Autodesk Inventor part; units mm, degrees
ref_plane "Work Plane1" through (0, 0, 60) normal (0, 0, -1) x (-1, 0, 0)
ref_plane "Work Plane2" through (0, 0, 192) normal (0, 0, -1) x (-1, 0, 0)
ref_plane "Work Plane3" through (0, -25.1413, 0) normal (-1, 0, 0) x (0, 0, 1)
sketch "Sketch1" plane through (0, 0, 0) normal (0, 0, 1) x (1, 0, 0)
  line L0 (0, 0) -> (-20.6965, 9.6509) construction
  line L1 (0, 0) -> (0, -60.6509) construction
  line L2 (0, 0) -> (-23.2307, -49.8183) construction
  line L3 (0, 0) -> (21.0241, 9.8037) construction
  line L4 (0, 0) -> (21.5225, -46.1553) construction
  line L5 (0, 0) -> (0, 48) construction
  arc A0 (-36, -19.5) -> (36, -19.5) centre (0, 48) ccw
  line L6 (-36, -19.5) -> (-36, -25.1413)
  line L7 (36, -19.5) -> (36, -25.1413)
  line L8 (-10, -40.5) -> (10, -40.5)
  line L9 (-10, -40.5) -> (-10, -37.2653)
  line L10 (10, -40.5) -> (10, -37.2653)
  line L11 (-17.6908, -33.679) -> (-16.0004, -30.0538)
  line L12 (-16.0004, -30.0538) -> (-12.7377, -31.5752)
  line L13 (-12.7377, -31.5752) -> (-14.4281, -35.2004)
  line L14 (14.4281, -35.2004) -> (12.7377, -31.5752)
  line L15 (12.7377, -31.5752) -> (16.0004, -30.0538)
  line L16 (16.0004, -30.0538) -> (17.6908, -33.679)
  line L17 (10, -37.2653) -> (14.4281, -35.2004)
  line L18 (17.6908, -33.679) -> (36, -25.1413)
  line L19 (-10, -37.2653) -> (-14.4281, -35.2004)
  line L20 (-17.6908, -33.679) -> (-36, -25.1413)
  dimension "d0" = 25
  dimension "d1" = 90
  dimension "d2" = 90
  dimension "d3" = 25
  dimension "d4" = 48
  dimension "d5" = 153
  dimension "d11" = 72
  dimension "d12" = 36
  dimension "d13" = 20
  dimension "d14" = 10
  dimension "d17" = 88.5
  dimension "d18" = 3.6
  dimension "d19" = 1.8
  dimension "d20" = 4
  dimension "d21" = 1.8
  dimension "d22" = 1.8
  dimension "d23" = 4
extrude "Extrusion1" add sketch "Sketch1" along normal blind 325
ref_plane "Work Plane1" through (0, 0, 60) normal (0, 0, -1) x (-1, 0, 0)
sketch "Sketch2" plane through (0, 0, 60) normal (0, 0, -1) x (-1, 0, 0)
  line L0 (14.4281, -35.2004) -> (12.7377, -31.5752)
  line L1 (12.7377, -31.5752) -> (16.0004, -30.0538)
  line L2 (14.4281, -35.2004) -> (10, -37.2653)
  line L3 (16.0004, -30.0538) -> (25.4652, -30.0538)
  line L4 (25.4652, -30.0538) -> (14.4281, -35.2004)
  line L5 (12.7377, -31.5752) -> (14.4281, -35.2004)
  line L6 (16.0004, -30.0538) -> (12.7377, -31.5752)
  line L7 (36, -25.1413) -> (17.6908, -33.679)
  line L8 (10, -40.5) -> (-10, -40.5)
  line L9 (-14.4281, -35.2004) -> (-12.7377, -31.5752)
  line L10 (-12.7377, -31.5752) -> (-16.0004, -30.0538)
  line L11 (-16.0004, -30.0538) -> (-25.4652, -30.0538)
  line L12 (-25.4652, -30.0538) -> (-14.4281, -35.2004)
  line L13 (-14.4281, -35.2004) -> (-12.7377, -31.5752)
  line L14 (-12.7377, -31.5752) -> (-16.0004, -30.0538)
  line L15 (-10, -37.2653) -> (-14.4281, -35.2004)
  line L16 (-17.6908, -33.679) -> (-36, -25.1413)
  point P0 (0, 0)
extrude "Extrusion2" cut sketch "Sketch2" against normal blind 72
ref_plane "Work Plane2" through (0, 0, 192) normal (0, 0, -1) x (-1, 0, 0)
sketch "Sketch3" plane through (0, 0, 192) normal (0, 0, -1) x (-1, 0, 0)
  line L0 (14.4281, -35.2004) -> (12.7377, -31.5752)
  line L1 (12.7377, -31.5752) -> (14.4281, -35.2004)
  line L2 (12.7377, -31.5752) -> (16.0004, -30.0538)
  line L3 (16.0004, -30.0538) -> (25.4652, -30.0538)
  line L4 (25.4652, -30.0538) -> (14.4281, -35.2004)
  line L5 (-14.4281, -35.2004) -> (-12.7377, -31.5752)
  line L6 (-12.7377, -31.5752) -> (-16.0004, -30.0538)
  line L7 (-16.0004, -30.0538) -> (-25.4652, -30.0538)
  line L8 (-25.4652, -30.0538) -> (-14.4281, -35.2004)
  line L9 (16.0004, -30.0538) -> (12.7377, -31.5752)
  line L10 (14.4281, -35.2004) -> (10, -37.2653)
  line L11 (-14.4281, -35.2004) -> (-12.7377, -31.5752)
  line L12 (-12.7377, -31.5752) -> (-16.0004, -30.0538)
  line L13 (-10, -37.2653) -> (-14.4281, -35.2004)
  line L14 (10, -40.5) -> (-10, -40.5)
  line L15 (36, -25.1413) -> (17.6908, -33.679)
  point P0 (0, 0)
extrude "Extrusion3" cut sketch "Sketch3" against normal blind 73
ref_plane "Work Plane3" through (0, -25.1413, 0) normal (-1, 0, 0) x (0, 0, 1)
sketch "Sketch5" plane through (0, -25.1413, 0) normal (-1, 0, 0) x (0, 0, 1)
  line L0 (0, -7.5587) -> (0, -3.3587)
  line L1 (68, -7.5587) -> (68, -15.3587)
  line L2 (68, -15.3587) -> (138.7768, -15.3587)
  line L3 (138.7768, -15.3587) -> (108, -5.3587)
  line L4 (108, -5.3587) -> (108, -3.3587)
  line L5 (0, -15.3587) -> (325, -15.3587)
  line L6 (246, -7.5587) -> (246, -15.3587)
  line L7 (246, -15.3587) -> (316.7768, -15.3587)
  line L8 (68, -7.5587) -> (0, -7.5587)
  line L9 (286, -3.3587) -> (286, -5.3587)
  line L10 (316.7768, -15.3587) -> (286, -5.3587)
  line L11 (0, -3.3587) -> (0, -0.3587)
  line L12 (0, -8.5377) -> (0, 0)
  line L13 (0, 5.6413) -> (325, 5.6413)
  line L14 (286, -0.3587) -> (286, -3.3587)
  line L15 (246, -7.5587) -> (148, -7.5587)
  line L16 (148, -7.5587) -> (148, -3.3587)
  line L17 (108, -0.3587) -> (108, -3.3587)
  line L18 (325, -3.3587) -> (0, -3.3587)
  line L19 (148, -3.3587) -> (148, -0.3587)
  line L20 (0, -3.3587) -> (108, -3.3587)
  line L21 (148, -3.3587) -> (286, -3.3587)
  line L22 (0, -0.3587) -> (108, -0.3587)
  line L23 (148, -0.3587) -> (286, -0.3587)
  point P0 (0, 25.1413)
  dimension "d51" = 4.2
  dimension "d52" = 0
  dimension "d53" = 68
  dimension "d54" = 2
  dimension "d56" = 40
  dimension "d59" = 246
  dimension "d64" = 18
  dimension "d65" = 2
  dimension "d68" = 3
  dimension "d69" = 40
  dimension "d84" = 178
  dimension "d94" = 18
  dimension "d96" = 40
extrude "Extrusion4" cut sketch "Sketch5" along normal mid plane 6.5 contours L0 L18 L4 L3 L2 L1 L8 | L11 L22 L17 L18 | L18 L9 L10 L5 L6 L15 L16 | L19 L23 L14 L18
sketch "Sketch6" plane through (-10, -40.5, 0) normal (0, -1, 0) x (1, 0, 0)
  line L0 (-49, 178) -> (79, 178) construction
  line L1 (10, 0) -> (10, 369) construction
  arc A0 (11, 159) -> (11, 169) centre (11, 164) ccw
  arc A1 (16, 183) -> (16, 173) centre (16, 178) ccw
  line L2 (11, 159) -> (11, 169)
  line L3 (16, 173) -> (16, 183)
  line L4 (11, 187) -> (11, 197)
  arc A2 (11, 187) -> (11, 197) centre (11, 192) ccw
  point P0 (4, 178)
  dimension "d70" = 178
  dimension "d85" = 1
  dimension "d86" = 5
  dimension "d87" = 5
  dimension "d88" = 6
  dimension "d89" = 5
  dimension "d90" = 1
  dimension "d91" = 14
  dimension "d92" = 14
extrude "Extrusion5" add sketch "Sketch6" along normal blind 7
equation "\"BendRadius\" = Thickness"
equation "\"BendReliefWidth\" = Thickness"
equation "\"BendReliefDepth\" = 0.5 * Thickness"
equation "\"CornerReliefSize\" = 4 * Thickness"
equation "\"MinimumRemnant\" = 2 * Thickness"
equation "\"TransitionRadius\" = BendRadius"
equation "\"JacobiRadiusSize\" = BendRadius"
equation "\"GapSize\" = Thickness"
properties part number "3213_Bed Holder" material "Acetal Resin, White"
Work out the finished part from the listing and answer in its coordinate system (mm). A direction names the side the tool comes from. Coordinates: 2 decimals unless noted, no trailing zeros. Write each loop counter-clockwise with the first axis right and the second up, starting at its lowest first coordinate (ties: lowest second). Pieces come first, ordered by that corner, then holes. Notation, with made-up numbers: M 53.25,-35 L 86.25,-35 A23 cw 86.25,0 Z; hole C 74.25,68.25 d11. An arc over 180 degrees is marked long. Write item = value, one per line.
1. The part is cut by section D-D (z = 164). Determine the outline of the cut face in (x, y), then the cut area to 3 significant figures.
Solution:
outline = M -36,-25.14 L -17.69,-33.68 L -16,-30.05 L -12.74,-31.58 L -14.43,-35.2 L -10,-37.27 L -10,-40.5 L 1,-40.5 L 1,-47.5 L 6,-47.5 L 6,-40.5 L 10,-40.5 L 10,-37.27 L 14.43,-35.2 L 12.74,-31.58 L 16,-30.05 L 17.69,-33.68 L 36,-25.14 L 36,-19.5 A76.5 cw 3.25,-28.43 L 3.25,-32.7 L -3.25,-32.7 L -3.25,-28.43 A76.5 cw -36,-19.5 Z
area = 570 mm2
2. The part is cut by section A-A (z = 39). Determine the outline of the cut face in (x, y), then the cut area to 3 significant figures.
Solution:
outline = M -36,-25.14 L -17.69,-33.68 L -16,-30.05 L -12.74,-31.58 L -14.43,-35.2 L -10,-37.27 L -10,-40.5 L 10,-40.5 L 10,-37.27 L 14.43,-35.2 L 12.74,-31.58 L 16,-30.05 L 17.69,-33.68 L 36,-25.14 L 36,-19.5 A76.5 cw 3.25,-28.43 L 3.25,-32.7 L -3.25,-32.7 L -3.25,-28.43 A76.5 cw -36,-19.5 Z
area = 535 mm2
3. The part is cut by section B-B (z = 101.5). Determine the outline of the cut face in (x, y).
Solution:
outline = M -36,-25.14 L -25.47,-30.05 L -16,-30.05 L -12.74,-31.58 L -14.43,-35.2 L -10,-37.27 L -10,-40.5 L -3.25,-40.5 L -3.25,-28.43 A76.5 cw -36,-19.5 Z; M 3.25,-40.5 L 10,-40.5 L 10,-37.27 L 14.43,-35.2 L 12.74,-31.58 L 16,-30.05 L 25.47,-30.05 L 36,-25.14 L 36,-19.5 A76.5 cw 3.25,-28.43 Z
4. The part is cut by section C-C (x = -6). Determine the outline of the cut face in (y, z), then the cut area to 3 significant figures.
Solution:
outline = M -40.5,0 L -28.26,0 L -28.26,325 L -40.5,325 Z
area = 3,980 mm2
5. Straight lines are drawn through the part: line 1 (Z direction, x = 20, y = -32); line 2 (X direction, y = -39.25, z = 122.5); line 3 (X direction, y = -32.25, z = 231.5). For each, find the intervals that lie inside material, in ascending order. Write a range as from..to.
Solution:
line_1 = 0..60, 132..192, 265..325
line_2 = -10..-3.25, 3.25..10
line_3 = -13.05..-3.25, 3.25..13.05
6. For faces 4 (the face through (-21, -30.054, 228)), 5 (the face through (21, -30.054, 228)), 6 (the face through (1, -44, 164)), determine the directions among +Z, -Z, +X, -X, +Y, -Y from which every point of the face is accessible in a straight line to the end or side of a thin tool.
Solution:
face_4 = -X, -Y
face_5 = +X, -Y
face_6 = +Z, -Z, -X, -Y
7. Flat-ended cylindrical pins translate along their axes: pin 1 (2 mm diameter, centred on x = 0, z = 217, fed in from +Y); pin 2 (6 mm diameter, centred on y = -29, z = 258, fed in from +X); pin 3 (10 mm diameter, centred on x = 21.5, z = 33, fed in from +Y); pin 4 (6 mm diameter, centred on x = 10, y = -36, fed in from -Z). Find the tip coordinate at first contact, or state that the pin passes through.
Solution:
pin_1 = -32.7
pin_2 = 34.16
pin_3 = -23.76
pin_4 = 0
8. Determine the mould class of faces 1 (the face through (-28.8, -28.5, 160.2)), 2 (the face through (0, -33, 0)), 3 (the face through (0.05, -35.57, 123.6)) for opening direction X: released by +X, released by -X, zero draft, split by the parting line, or undercut.
Solution:
face_1 = released by -X
face_2 = zero draft
face_3 = undercut
